Build history of the part. All positions in model axes, mm. Face numbers are marked on the shaded views. A direction names the side the tool comes from. Coordinates: 2 decimals unless noted, no trailing zeros. Order: outer loops, then holes, each group sorted by start corner. A loop starts at its lowest first (then second) coordinate and runs counter-clockwise, first axis right, second up. Notation, with made-up numbers: M -34,9.25 L 11,9.25 A20 ccw 11,42.25 Z; hole C 83,30.5 d5. An arc over 180 degrees is marked long. Write item = value, one per line. Start each with the question number.
Q1. Band-saw the part on C-C on z = 31.5. Write the cut outline in (x, y).
Q2. Pin check, flat tips, straight feed: P1, Ø0.9, axis at y = 22.5, z = 29.5, coming from the +X side; P2, Ø3.5, axis at x = -1.5, z = 28, coming from the +Y side; P3, Ø3.5, axis at y = 22.5, z = 31, coming from the -X side; P4, Ø2.5, axis at y = -22.5, z = 30, coming from the +X side. Stop position of each tip, or through.
Q3. Drill centre lines: probe 1 along Z at (x, y) = (-3.85, 0); probe 2 along Y at (x, z) = (1.5, 26); probe 3 along Y at (x, z) = (0, 2.25). Where is each one in solid material? Low to high.
Q4. Pull direction Y, two halves, no side cores. Call the marked faces 1, 2 and 3: released by +Y, released by -Y, zero draft, split by the parting line, or undercut.
Q5. Band-saw the part on D-D on y = 0. Write the cut outline in (x, z).
Q6. 3-axis set-ups, long thin cutter, end or side, ignore diameter. For the marked faces 4 and 5: which of +Z, -Z, +X, -X, +Y, -Y reach the whole face in a straight line?
Q7. Band-saw the part on A-A on z = 25. Write the cut outline in (x, y).
Q8. Band-saw the part on B-B on x = 0. Write the cut outline in (y, z), plus the area to 3 significant figures.
Autodesk Inventor part; units mm, degrees
ref_plane "YZ Plane" through (0, 0, 0) normal (1, 0, 0) x (0, 1, 0)
ref_plane "XZ Plane" through (0, 0, 0) normal (0, 1, 0) x (-1, 0, 0)
ref_plane "XY Plane" through (0, 0, 0) normal (0, 0, 1) x (1, 0, 0)
sketch "Sketch1" plane through (0, 0, 0) normal (0, 0, 1) x (1, 0, 0)
  arc A0 (-9.2513, -12.8456) -> (-7.7191, -13.7193) centre (-8.2517, -12.873) ccw
  line L0 (-7.7191, -13.7193) -> (-1.0653, -9.532)
  arc A1 (1.0653, -9.532) -> (-1.0653, -9.532) centre (0, -11.2247) ccw
  line L1 (1.0653, -9.532) -> (7.7191, -13.7193)
  arc A2 (7.7191, -13.7193) -> (9.2513, -12.8456) centre (8.2517, -12.873) ccw
  arc A3 (12.8456, -9.2513) -> (9.2513, -12.8456) centre (12.75, -12.75) ccw
  arc A4 (12.8456, -9.2513) -> (13.7193, -7.7191) centre (12.873, -8.2517) ccw
  line L2 (13.7193, -7.7191) -> (9.532, -1.0653)
  arc A5 (9.532, 1.0653) -> (9.532, -1.0653) centre (11.2247, 0) ccw
  line L3 (9.532, 1.0653) -> (13.7385, 7.7495)
  line L4 (7.7677, 13.7499) -> (1.0653, 9.532)
  arc A6 (-1.0653, 9.532) -> (1.0653, 9.532) centre (0, 11.2247) ccw
  line L5 (-1.0653, 9.532) -> (-7.7191, 13.7193)
  arc A7 (-7.7191, 13.7193) -> (-9.2513, 12.8456) centre (-8.2517, 12.873) ccw
  arc A8 (-12.8456, 9.2513) -> (-9.2513, 12.8456) centre (-12.75, 12.75) ccw
  arc A9 (-12.8456, 9.2513) -> (-13.7193, 7.7191) centre (-12.873, 8.2517) ccw
  line L6 (-13.7193, 7.7191) -> (-9.532, 1.0653)
  arc A10 (-9.532, -1.0653) -> (-9.532, 1.0653) centre (-11.2247, 0) ccw
  line L7 (-9.532, -1.0653) -> (-13.7193, -7.7191)
  arc A11 (-13.7193, -7.7191) -> (-12.8456, -9.2513) centre (-12.873, -8.2517) ccw
  arc A12 (-9.2513, -12.8456) -> (-12.8456, -9.2513) centre (-12.75, -12.75) ccw
  circle A13 centre (0, 0) radius 2.5
  circle A14 centre (0, 0) radius 2
  circle A15 centre (0, 0) radius 2.1
  line L8 (2.8, -24.1) -> (-2.8, -24.1)
  line L9 (-2.8, 24.1) -> (2.8, 24.1)
  line L10 (2.8, -24.1) -> (7.5, -2.9)
  line L11 (7.5, 2.9) -> (2.8, 24.1)
  line L12 (-2.8, 24.1) -> (-7.5, 2.9)
  line L13 (-7.5, -2.9) -> (-2.8, -24.1)
  line L14 (7.5, -2.9) -> (7.5, 2.9)
  line L15 (-7.5, 2.9) -> (-7.5, -2.9)
  line L16 (7.5, -2.9) -> (-7.5, -2.9) construction
  line L17 (-7.5, 2.9) -> (7.5, 2.9) construction
  line L18 (2.8, -24.1) -> (2.8, 24.1) construction
  line L19 (-2.8, 24.1) -> (-2.8, -24.1) construction
  line L20 (7.5, 0) -> (0, 0) construction
  line L21 (0, 0) -> (-7.5, 0) construction
  line L22 (-2.5, -2.9) -> (-2.5, 2.9) construction
  arc A16 (9.3, 12.8764) -> (7.7677, 13.7499) centre (8.3003, 12.9036) ccw
  arc A17 (13.7385, 7.7495) -> (12.8714, 9.2819) centre (12.8922, 8.2822) ccw
  arc A18 (9.3, 12.8764) -> (12.8714, 9.2819) centre (12.7987, 12.7812) ccw
  dimension "d0" = 0.1
  dimension "d5" = 48.2
  dimension "d6" = 5.6
  dimension "d7" = 5
  dimension "d8" = 5.8
extrude "Extrusion1" add sketch "Sketch1" along normal blind 6.8 contours L13 L15 L12 L5 A6 L4 L11 L14 L10 L1 A1 L0 | L0 A1 L1 L10 L8 L13 | L12 L9 L11 L4 A6 L5
sketch "Sketch2" plane through (-7.5, -2.9, 0) normal (-1, 0, 0) x (0, 0, 1)
  line L0 (0, 5.8) -> (0, 0)
  line L1 (0, 0) -> (6.8, 0)
  line L2 (6.8, 5.8) -> (6.8, 0)
  line L3 (0, 5.8) -> (6.8, 5.8)
  circle A0 centre (3.4, 2.9) radius 1.6
  point P0 (0, 2.9)
  dimension "d9" = 3.2
extrude "Extrusion2" cut sketch "Sketch2" against normal blind 7.4875 contours A0
sketch "Sketch3" plane through (0, 0, 6.8) normal (0, 0, 1) x (1, 0, 0)
  line L0 (7.5, 2.9) -> (2.8, 24.1)
  line L1 (2.8, 24.1) -> (-2.8, 24.1)
  line L2 (-2.8, 24.1) -> (-7.5, 2.9)
  line L3 (-7.5, 2.9) -> (-7.5, -2.9)
  line L4 (-7.5, -2.9) -> (-2.8, -24.1)
  line L5 (-2.8, -24.1) -> (2.8, -24.1)
  line L6 (2.8, -24.1) -> (7.5, -2.9)
  line L7 (7.5, -2.9) -> (7.5, 2.9)
  circle A0 centre (0, 0) radius 2.5
  line L8 (3.4651, -21.1) -> (-3.4651, -21.1)
  line L9 (-3.4651, 21.1) -> (3.4651, 21.1)
  point P0 (0, 0)
  dimension "d19" = 3
  dimension "d20" = 3
extrude "Extrusion3" add sketch "Sketch3" along normal blind 29.1 contours L9 L2 L1 L0 | L6 L5 L4 L8
sketch "Sketch4" plane through (-2.8, 24.1, 0) normal (0, 1, 0) x (1, 0, 0)
  line L0 (5.6, 0) -> (0, 0) construction
  line L1 (0, 0) -> (0, -35.9) construction
  line L2 (5.6, 0) -> (5.6, -35.9) construction
  line L3 (5.6, -35.9) -> (0, -35.9)
  line L4 (6.2651, -35.9) -> (-0.6651, -35.9) construction
  line L5 (2.8, -35.9) -> (2.8, 0) construction
  line L6 (5.6, -32.9) -> (0, -32.9) construction
  line L7 (4.5, -32.9) -> (1.1, -32.9)
  line L8 (1.1, -32.9) -> (1.1, -26.1)
  line L9 (1.1, -26.1) -> (4.5, -26.1)
  line L10 (4.5, -26.1) -> (4.5, -32.9)
  dimension "d23" = 3
  dimension "d25" = 3.4
  dimension "d26" = 6.8
extrude "Extrusion4" cut sketch "Sketch4" against normal through all
fillet "Fillet1" radius 2 2 edges at (0, -21.1, 6.8) (0, 21.1, 6.8)
equation "\"d20\" = d19"
equation "\"d26\" = 2 * d25"
properties part number "TurretPressFit"
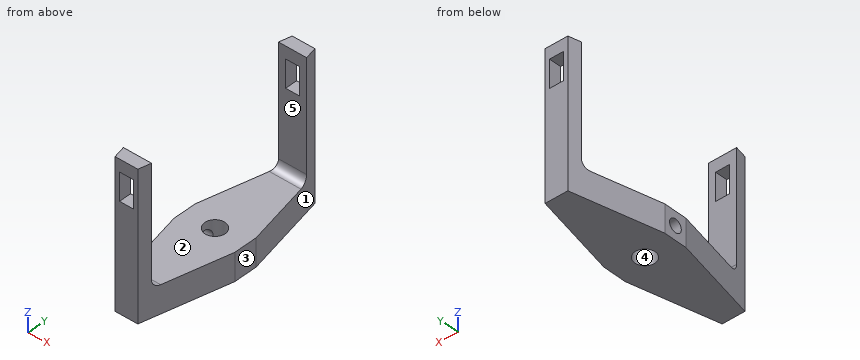
Recorded:
q1.outline = M -3.47,-21.1 L -2.8,-24.1 L -1.7,-24.1 L -1.7,-21.1 Z; M -3.47,21.1 L -1.7,21.1 L -1.7,24.1 L -2.8,24.1 Z; M 1.7,-24.1 L 2.8,-24.1 L 3.47,-21.1 L 1.7,-21.1 Z; M 1.7,21.1 L 3.47,21.1 L 2.8,24.1 L 1.7,24.1 Z
q2.P1 = 3.25
q2.P2 = 24.1
q2.P3 = -3.47
q2.P4 = 3.43
q3.probe_1 = 0 to 1.8, 5 to 6.8
q3.probe_2 = -24.1 to -21.1, 21.1 to 24.1
q3.probe_3 = -24.1 to -2.5, 2.5 to 24.1
q4.face_1 = released by +Y
q4.face_2 = undercut
q4.face_3 = zero draft
q5.outline = M -7.5,0 L -2.5,0 L -2.5,1.8 L -7.5,1.8 Z; M -7.5,5 L -2.5,5 L -2.5,6.8 L -7.5,6.8 Z; M 2.5,0 L 7.5,0 L 7.5,6.8 L 2.5,6.8 Z
q6.face_4 = +Z, -Z
q6.face_5 = +Z, +X, -X
q7.outline = M -3.47,-21.1 L -2.8,-24.1 L 2.8,-24.1 L 3.47,-21.1 Z; M -3.47,21.1 L 3.47,21.1 L 2.8,24.1 L -2.8,24.1 Z
q8.outline = M -24.1,0 L -2.5,0 L -2.5,6.8 L -19.1,6.8 A2 cw -21.1,8.8 L -21.1,26.1 L -24.1,26.1 Z; M -24.1,32.9 L -21.1,32.9 L -21.1,35.9 L -24.1,35.9 Z; M 2.5,0 L 24.1,0 L 24.1,26.1 L 21.1,26.1 L 21.1,8.8 A2 cw 19.1,6.8 L 2.5,6.8 Z; M 21.1,32.9 L 24.1,32.9 L 24.1,35.9 L 21.1,35.9 Z
q8.area = 429 mm2
